```python
from build123d import *

# Parameters (mm, degrees)
SALIENTE_EXTRUIR1_DEPTH = 91
CROQUIS3_W              = 21.106040847
CROQUIS3_H              = 4.330702007
CROQUIS3_W_2            = 30.122472971
CROQUIS3_H_2            = 14
CORTAR_EXTRUIR2_DEPTH   = 91
CROQUIS4_W              = 22.111814678
CROQUIS4_H              = 2.5
CORTAR_EXTRUIR3_DEPTH   = 10
CORTAR_EXTRUIR4_DEPTH   = 10


with BuildPart() as part:
    # Croquis1 → Saliente-Extruir1 (new body)
    with BuildSketch(Plane.XY):
        Polygon((-53.839851527, -4.678337985), (-53.839851527, -5.641142559), (84.70895538, -5.641142559), (84.804732082, -4.678337985), align=None)
    extrude(amount=SALIENTE_EXTRUIR1_DEPTH)

    # Croquis3 → Cortar-Extruir2 (cut)
    with BuildSketch(Plane(origin=(0, -4.678337985, 0), x_dir=(1, 0, 0), z_dir=(0, 1, 0))):
        with Locations((16.385259295, -87.334648996)):
            Rectangle(CROQUIS3_W, CROQUIS3_H)
        with Locations((77.75415389, -9.5)):
            Rectangle(CROQUIS3_W_2, CROQUIS3_H_2)
        with Locations((77.75415389, -87.5)):
            Rectangle(CROQUIS3_W_2, CROQUIS3_H_2)
    extrude(amount=-CORTAR_EXTRUIR2_DEPTH, mode=Mode.SUBTRACT)

    # Croquis4 → Cortar-Extruir3 (cut)
    with BuildSketch(Plane(origin=(0, -4.678337985, 0), x_dir=(1, 0, 0), z_dir=(0, 1, 0))):
        with Locations((73.748824743, -1.25)):
            Rectangle(CROQUIS4_W, CROQUIS4_H)
    extrude(amount=-CORTAR_EXTRUIR3_DEPTH, mode=Mode.SUBTRACT)

    # Croquis5 → Cortar-Extruir4 (cut)
    with BuildSketch(Plane(origin=(0, -4.678337985, 0), x_dir=(1, 0, 0), z_dir=(0, 1, 0))):
        Polygon((5.832238872, -89.5), (5.832238872, -91), (26.950480476, -91), (26.938279719, -89.5), align=None)
    extrude(amount=-CORTAR_EXTRUIR4_DEPTH, mode=Mode.SUBTRACT)


solid = part.part
```
Read the model definition and answer for the solid it produces. Units are mm, in the model's axes. Coordinates: 2 decimals unless noted, no trailing zeros. Loops run counter-clockwise (first coordinate to the right, second up) from the corner with the lowest first, then second, coordinate; pieces in that order, holes last. Notation, with made-up numbers: (7, 36) -> (42, 36) arc R18 cw to (42, 54) -> close; hole circle Ø9 at (20, -38). An arc over 180 degrees is marked (long way). Return JSON: item names as keys, results as strings.
Item 1: Flat-ended cylindrical pins translate along their axes: P1, Ø0.5, axis at x = 76.5, y = -5, coming from the -Z side; P2, Ø0.5, axis at y = -5, z = 85, coming from the +X side. Find the tip coordinate at first contact, or state that the pin passes through.
Answers:
{"P1": "stops at z = 16.5", "P2": "stops at x = 62.69"}
Item 2: Find section B-B (x = 8). Determine the outline of the cut face in (y, z).
Answers:
{"outline": "(-5.64, 0) -> (-4.68, 0) -> (-4.68, 85.17) -> (-5.64, 85.17) -> close"}
Item 3: Find the intervals of material crossed by probe 1 along X at (y, z) = (-4.85, 29); probe 2 along X at (y, z) = (-4.75, 85); probe 3 along Z at (x, y) = (7.5, -5.4), in increasing order.
Answers:
{"probe 1": "x = -53.84 to 84.79", "probe 2": "x = -53.84 to 62.69", "probe 3": "z = 0 to 85.17"}
Item 4: Find section A-A (y = -5). Determine the outline of the cut face in (x, z), plus the area to 3 significant figures.
Answers:
{"outline": "(-53.84, 0) -> (62.69, 0) -> (62.69, 16.5) -> (84.77, 16.5) -> (84.77, 80.5) -> (62.69, 80.5) -> (62.69, 91) -> (26.95, 91) -> (26.94, 89.5) -> (26.94, 85.17) -> (5.83, 85.17) -> (5.83, 91) -> (-53.84, 91) -> close", "area": "11,900 mm2"}
